from build123d import *

# Parameters (mm, degrees)
ESQUISSE1_W                = 20
ESQUISSE1_H                = 18
MAIN_EXTRUSION_DEPTH       = 30
MAIN_RIDING_HOLE_DEPTH     = 31
ESQUISSE4_R                = 2.25
TRACTORHOLE_DEPTH          = 8
BOSS_EXTRU_1_DEPTH         = 4.5
R_P_TITION_LIN_AIRE1_COUNT = 6
R_P_TITION_LIN_AIRE1_PITCH = 4.71238898


with BuildPart() as part:
    # Esquisse1 → Main Extrusion (new body)
    with BuildSketch(Plane.XY):
        Rectangle(ESQUISSE1_W, ESQUISSE1_H)
    extrude(amount=MAIN_EXTRUSION_DEPTH)

    # Esquisse3 → Main Riding Hole (cut, through all)
    with BuildSketch(Plane(origin=(0, 0, 0), x_dir=(-1, 0, 0), z_dir=(0, 0, -1))):
        Polygon((-5.2, 4.4), (-5.2, 0.6), (-4.2, 0.6), (-4.2, -2.2), (-5.2, -2.2), (-5.2, -6), (-1.4, -6), (-1.4, -5), (1.4, -5), (1.4, -6), (5.2, -6), (5.2, -2.2), (4.2, -2.2), (4.2, 0.6), (5.2, 0.6), (5.2, 4.4), (1.4, 4.4), (1.4, 3.4), (-1.4, 3.4), (-1.4, 4.4), align=None)
    extrude(amount=-MAIN_RIDING_HOLE_DEPTH, mode=Mode.SUBTRACT)

    # Esquisse4 → TractorHole (cut)
    with BuildSketch(Plane.ZY.offset(10)):
        with Locations((5, -0.8)):
            Circle(ESQUISSE4_R)
    tractorhole = extrude(amount=-TRACTORHOLE_DEPTH, mode=Mode.SUBTRACT)

    # TractorHoleSymetry: TractorHole across plane
    add(tractorhole.mirror(Plane(origin=(0, 0, 0), x_dir=(0, 0, 1), z_dir=(1, 0, 0))), mode=Mode.SUBTRACT)

    # Esquisse8 → Boss.-Extru.1 (add, symmetric)
    with BuildSketch(Plane(origin=(0, 0, 0), x_dir=(0, 0, -1), z_dir=(1, 0, 0))):
        Polygon((-3.721082869, 9), (-2.492683328, 12.375), (-1.228399541, 12.375), (0, 9), align=None)
    boss_extru_1 = extrude(amount=BOSS_EXTRU_1_DEPTH, both=True)

    # Répétition linéaire1: Boss.-Extru.1 ×6
    with Locations(*[(0, 0, i * R_P_TITION_LIN_AIRE1_PITCH) for i in range(1, R_P_TITION_LIN_AIRE1_COUNT)]):
        add(boss_extru_1)


solid = part.part
Geometry: final body of the model. Coordinates: model frame, mm. A direction names the side the tool comes from. Round coordinates to 2 decimals unless told otherwise and drop trailing zeros. Loops run counter-clockwise (first coordinate to the right, second up) from the corner with the lowest first, then second, coordinate; pieces in that order, holes last. Notation, with made-up numbers: M 79.25,89.25 L 119.25,89.25 A9 ccw 119.25,94.25 Z; hole C 24,0 d9. An arc over 180 degrees is marked long. One line per question, with ' | ' between items.
(1) Material intervals for line 1 along Y through (x, z) = (-8.1, 5); line 2 along Z through (x, y) = (7.6, -0.8); line 3 along X through (y, z) = (3, 11.25), sorted ascending. Write a range as from..to.
Check result:
line 1: y = -9..-3.05, 1.45..9 | line 2: z = 0..2.75, 7.25..30 | line 3: x = -10..-5.2, 5.2..10
(2) Contact query for flat-ended pins moving along their axis: P1, Ø3.5, axis at y = 11, z = 20.5, coming from the +X side; P2, Ø0.8, axis at x = -5, z = 21.5, coming from the +Y side. Output: stop coordinate, or through.
Check result:
P1: stops at x = 4.5 | P2: stops at y = 9
(3) Cut plane C-C on x = -7.5. Return the cut outline in (y, z).
Check result:
outline: M -9,0 L 9,0 L 9,30 L -9,30 Z; hole C -0.8,5 d4.5
(4) Pull-direction query (X, two-part tool) for faces 1 (the flat face through (-4.5, 10, 25)), 2 (the flat face through (0, 12.375, 25)), 3 (the flat face through (4.5, 10, 11)), 4 (the flat face through (-5.2, 2, 15)); classes: +X half, -X half, draft (parallel to the pull), parting line (faces both ways), or undercut.
Check result:
face 1: -X half | face 2: draft | face 3: +X half | face 4: undercut
(5) Cut plane A-A on y = 2.5. Return the cut outline in (x, z).
Check result:
outline: M -10,0 L -5.2,0 L -5.2,30 L -10,30 Z; M 5.2,0 L 10,0 L 10,30 L 5.2,30 Z
(6) Cut plane B-B on y = -0.8. Return the cut outline in (x, z), plus the area to 3 significant figures.
Check result:
outline: M -10,0 L -4.2,0 L -4.2,2.75 L -10,2.75 Z; M -10,7.25 L -4.2,7.25 L -4.2,30 L -10,30 Z; M 4.2,0 L 10,0 L 10,2.75 L 4.2,2.75 Z; M 4.2,7.25 L 10,7.25 L 10,30 L 4.2,30 Z | area: 296 mm2
(7) Access query for faces 5 (the flat face through (0.06, 10.66, 12.54)), 6 (the flat face through (4.5, 10, 16)), 7 (the flat face through (0, 3.4, 15)), 8 (the flat face through (-4.5, 10, 11)), 9 (the flat face through (0, 12.375, 16)). Directions: +Z, -Z, +X, -X, +Y, -Y. A direction counts if a zero-diameter tool reaches every point of the face in a straight line with its end or side. Return the directions, or none.
Check result:
face 5: +X, -X, +Y | face 6: +Z, -Z, +X, +Y | face 7: +Z, -Z | face 8: +Z, -Z, -X, +Y | face 9: +Z, -Z, +X, -X, +Y
